Source: CAD feature listing. Evaluate the final solid. Frame: model axes, mm. A direction names the side the tool comes from. Give positions to 0.01 mm unless a question says otherwise; leave off trailing zeros. Loops run counter-clockwise (first coordinate to the right, second up) from the corner with the lowest first, then second, coordinate; pieces in that order, holes last. Notation, with made-up numbers: M -13,-17.75 L 0,-17.75 A20 ccw 0,2.25 Z; hole C 11,53 d9. An arc over 180 degrees is marked long. Put each result on its own line as item: value.
from build123d import *

# Parameters (mm, degrees)
SKETCH1_R           = 15
BOSS_EXTRUDE1_DEPTH = 20
SKETCH2_W           = 40
SKETCH2_H           = 50
BOSS_EXTRUDE2_DEPTH = 110
SKETCH3_W           = 18
SKETCH3_H           = 150
CUT_EXTRUDE1_DEPTH  = 139.293166859
SKETCH4_R           = 4
CUT_EXTRUDE2_DEPTH  = 141.712472795
CHAMFER1_SIZE       = 10


with BuildPart() as part:
    # Sketch1 → Boss-Extrude1 (new body)
    with BuildSketch(Plane(origin=(0, 0, 0), x_dir=(1, 0, 0), z_dir=(0, 1, 0))):
        with Locations(Location((0, 0, 0), (0, 0, 270))):
            Circle(SKETCH1_R)
    extrude(amount=BOSS_EXTRUDE1_DEPTH)

    # Sketch2 → Boss-Extrude2 (add)
    with BuildSketch(Plane(origin=(0, 20, 0), x_dir=(1, 0, 0), z_dir=(0, 1, 0))):
        Rectangle(SKETCH2_W, SKETCH2_H)
    extrude(amount=BOSS_EXTRUDE2_DEPTH)

    # Sketch3 → Cut-Extrude1 (cut, through all)
    with BuildSketch(Plane(origin=(20, 0, 0), x_dir=(0, 0, -1), z_dir=(1, 0, 0))):
        with Locations((0, 130)):
            Rectangle(SKETCH3_W, SKETCH3_H)
    extrude(amount=-CUT_EXTRUDE1_DEPTH, mode=Mode.SUBTRACT)

    # Sketch4 → Cut-Extrude2 (cut, through all)
    with BuildSketch(Plane(origin=(0, 0, -25), x_dir=(-1, 0, 0), z_dir=(0, 0, -1))):
        with Locations((0, 116)):
            Circle(SKETCH4_R)
    extrude(amount=-CUT_EXTRUDE2_DEPTH, mode=Mode.SUBTRACT)

    # Chamfer1
    chamfer1_edges = [part.edges().sort_by_distance(p)[0] for p in [
        (20, 130, -17),
        (-20, 130, 17),
        (20, 130, 17),
        (-20, 130, -17),
    ]]
    chamfer(chamfer1_edges, length=CHAMFER1_SIZE)


solid = part.part
1. Section query C-C (z = 0). Output: boundary loops of the cut face in (x, y).
Found:
outline: M -20,20 L -15,20 L -15,0 L 15,0 L 15,20 L 20,20 L 20,55 L -20,55 Z
2. Access query for faces 1 (the flat face through (-15, 125, 17)), 2 (the cylindrical face through (0.66, 9.86, -14.985)), 3 (the flat face through (0, 92, -9)). Directions: +Z, -Z, +X, -X, +Y, -Y. A direction counts if a zero-diameter tool reaches every point of the face in a straight line with its end or side. Return the directions, or none.
Found:
face 1: +Z, -Z, -X, +Y
face 2: -Y
face 3: +X, -X, +Y
3. Material intervals for line 1 (Y direction, x = 0, z = -18.75); line 2 (Z direction, x = 9, y = 107); line 3 (X direction, y = 9, z = 0), sorted ascending. Write a range as from..to.
Found:
line 1: 20..112, 120..130
line 2: -25..-9, 9..25
line 3: -15..15
4. Contact query for a flat-ended pin moving along its axis: P1, Ø1.5, axis at x = -14.5, z = -9.5, coming from the +Y side. Output: stop coordinate, or through.
Found:
P1: y = 126.25
5. Section query A-A (y = 116). Output: boundary loops of the cut face in (x, z).
Found:
outline: M -20,-25 L -4,-25 L -4,-9 L -20,-9 Z; M -20,9 L -4,9 L -4,25 L -20,25 Z; M 4,-25 L 20,-25 L 20,-9 L 4,-9 Z; M 4,9 L 20,9 L 20,25 L 4,25 Z
6. Section query D-D (y = 95). Output: boundary loops of the cut face in (x, z), plus the area to 3 significant figures.
Found:
outline: M -20,-25 L 20,-25 L 20,-9 L -20,-9 Z; M -20,9 L 20,9 L 20,25 L -20,25 Z
area: 1,280 mm^2
7. Draft query along Z for faces 4 (the flat face through (0, 55, 0)), 5 (the flat face through (0, 130, -17)), 6 (the flat face through (0, 74, -25)), 7 (the flat face through (0, 92, 9)). Return one class per face: pulls with the +Z half, pulls with the -Z half, needs draft (parallel to the pull), parting line crosses it, or undercut.
Found:
face 4: undercut
face 5: needs draft
face 6: pulls with the -Z half
face 7: undercut
8. Section query B-B (x = 0). Output: boundary loops of the cut face in (y, z), plus the area to 3 significant figures.
Found:
outline: M 0,-15 L 20,-15 L 20,-25 L 112,-25 L 112,-9 L 55,-9 L 55,9 L 112,9 L 112,25 L 20,25 L 20,15 L 0,15 Z; M 120,-25 L 130,-25 L 130,-9 L 120,-9 Z; M 120,9 L 130,9 L 130,25 L 120,25 Z
area: 4,490 mm^2
